Source: three-view drawing plus pictorial views. Frame: mm from the lowest corner of the part. A direction names the side the tool comes from. Round coordinates to 2 decimals unless told otherwise and drop trailing zeros. Write each loop counter-clockwise with the first axis right and the second up, starting at its lowest first coordinate (ties: lowest second). Pieces come first, ordered by that corner, then holes. Notation, with made-up numbers: (64, 83) -> (98, 83) arc R38 cw to (98, 122) -> close; hole circle Ø7 at (49, 64.25). An arc over 180 degrees is marked (long way). Put each result on its own line as item: value.
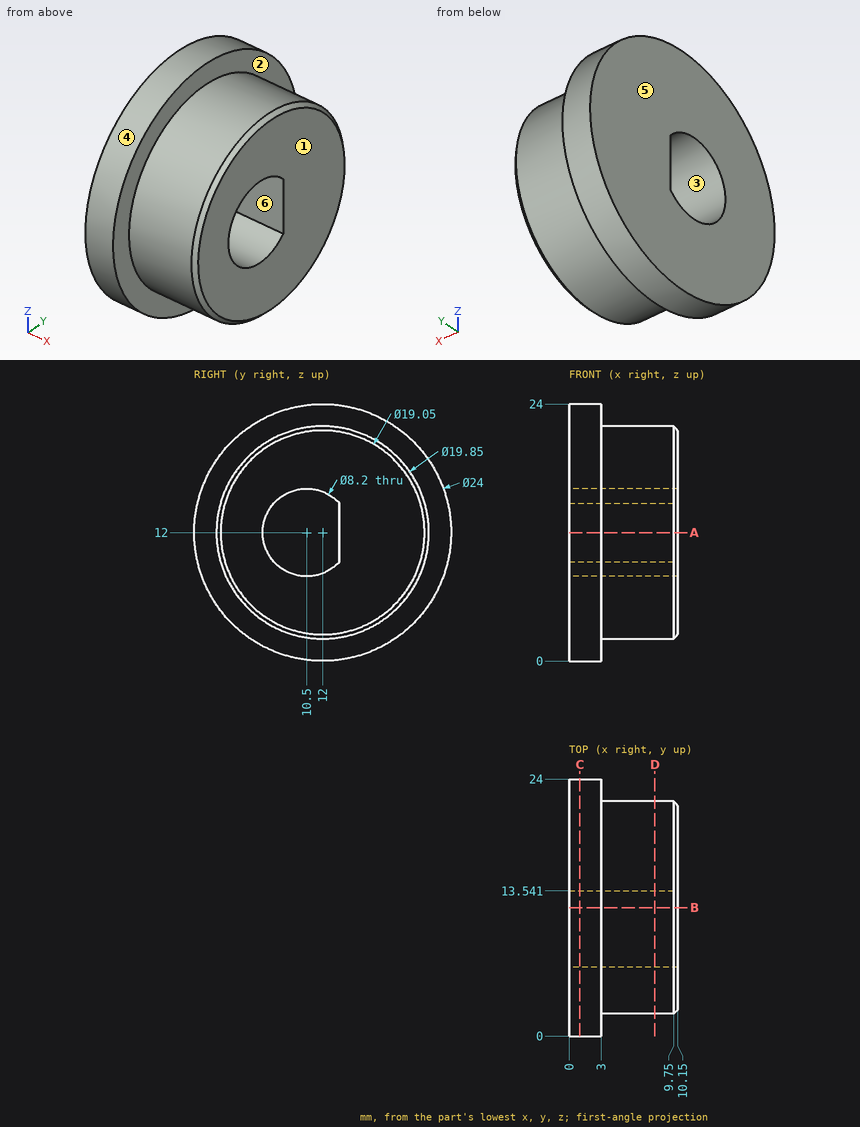
Q1. Draft query along Y for the marked faces 3, 4, 5 and 6. Return one class per face: +Y half, -Y half, draft (parallel to the pull), parting line (faces both ways), or undercut.
Ans:
face 3: undercut
face 4: parting line
face 5: draft
face 6: undercut
Q2. Cut plane D-D on x = 8. Output: boundary loops of the cut face in (y, z) (3 decimals).
Ans:
outline: circle Ø19.85 at (12, 12); hole (13.541, 9.25) -> (13.541, 14.75) arc R4.1 ccw (long way) to start
Q3. Material intervals for line 1 (Y direction, x = 2.5, z = 12); line 2 (Y direction, x = 5.25, z = 12) (3 decimals); line 3 (Z direction, x = 4.5, y = 10.5), sorted ascending. Write a range as [from, to].
Ans:
line 1: y = [0, 6.4], [13.54, 24]
line 2: y = [2.075, 6.4], [13.541, 21.925]
line 3: z = [2.19, 7.9], [16.1, 21.81]
Q4. Cut plane A-A on z = 12. Output: boundary loops of the cut face in (x, y) (3 decimals).
Ans:
outline: (0, 0) -> (3, 0) -> (3, 2.075) -> (9.75, 2.075) -> (10.15, 2.475) -> (10.15, 6.4) -> (0, 6.4) -> close; (0, 13.541) -> (10.15, 13.541) -> (10.15, 21.525) -> (9.75, 21.925) -> (3, 21.925) -> (3, 24) -> (0, 24) -> close
Q5. Pin query (flat end, axial travel): pin 1 (1.6 mm diameter, centred on x = 5.5, z = 11, fed in from -Y); pin 2 (1.5 mm diameter, centred on x = 8.5, z = 14, fed in from -Y). Return the tip coordinate at first contact, or that it passes through.
Ans:
pin 1: stops at y = 2.08
pin 2: stops at y = 2.15
Q6. Reachability of the marked faces 1 and 2 from +Z, -Z, +X, -X, +Y, -Y: full face, straight path, thin tool, end or side. Return the list, or none.
Ans:
face 1: +Z, -Z, +X, +Y, -Y
face 2: +X
Q7. Cut plane B-B on y = 12. Output: boundary loops of the cut face in (x, z) (3 decimals), and give its area (3 significant figures).
Ans:
outline: (0, 0) -> (3, 0) -> (3, 2.075) -> (9.75, 2.075) -> (10.15, 2.475) -> (10.15, 8.184) -> (0, 8.184) -> close; (0, 15.816) -> (10.15, 15.816) -> (10.15, 21.525) -> (9.75, 21.925) -> (3, 21.925) -> (3, 24) -> (0, 24) -> close
area: 136 mm^2
Q8. Cut plane C-C on x = 1. Output: boundary loops of the cut face in (y, z).
Ans:
outline: circle Ø24 at (12, 12); hole (13.54, 9.25) -> (13.54, 14.75) arc R4.1 ccw (long way) to start
